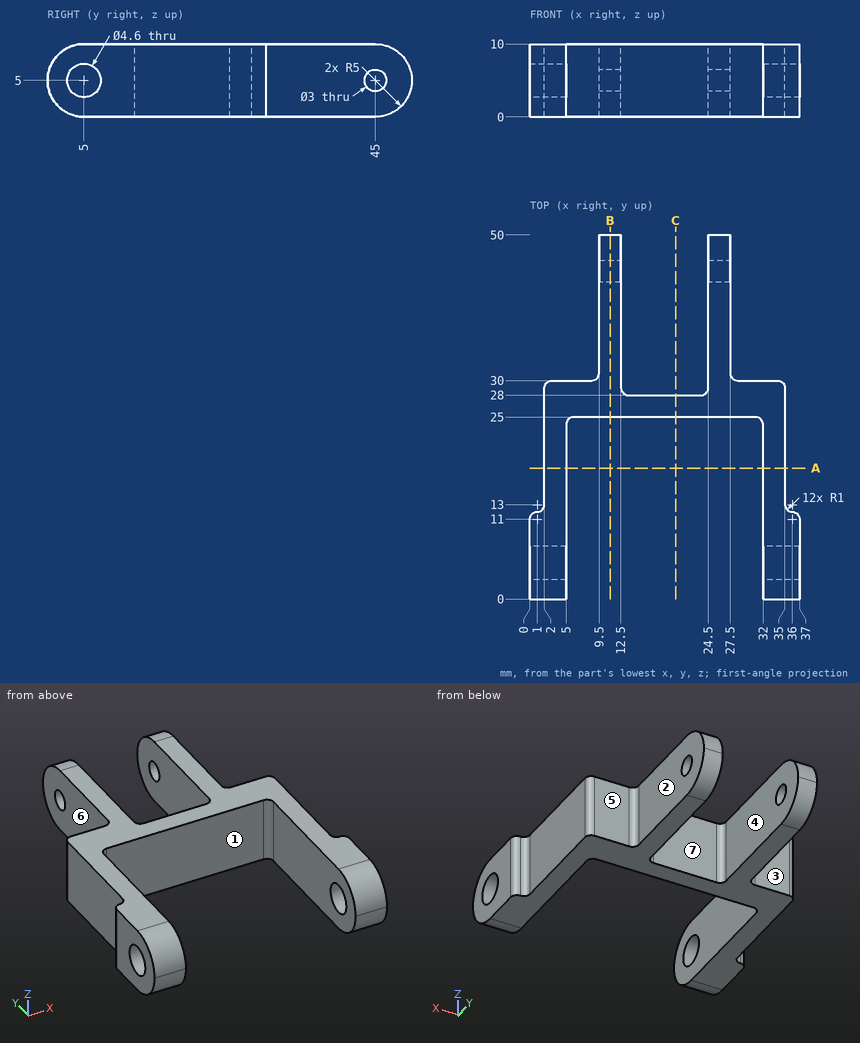
Here's the drawing with two shaded views (mm, measured from the low corner). I have some questions. A direction names the side the tool comes from. Give positions to 0.01 mm unless a question says otherwise; leave off trailing zeros. Write each loop counter-clockwise with the first axis right and the second up, starting at its lowest first coordinate (ties: lowest second). Pieces come first, ordered by that corner, then holes. Notation, with made-up numbers: (45, -25.5) - (49, -25.5) arc R28 ccw to (49, -0.5) - close; hole circle Ø5 at (-19, 34.25). An arc over 180 degrees is marked (long way). Write item = value, one per line. Start each with the question number.
1. On a 3-axis mill with a long thin cutter (end or side, diameter ignored), from which of +Z, -Z, +X, -X, +Y, -Y can I reach the whole of each face in a straight line? I mean the marked faces 1, 2, 3 and 4. Say none if no direction works.
2. Imagine slicing it at A-A (y = 18). Please give me the cut outline in (x, z).
3. Thinking about a two-plate mould opening in X: for the marked faces 5, 6 and 7, which applies, released by +X, released by -X, zero draft, split by the parting line, or undercut?
4. For pin 1 (3 mm diameter, centred on x = 6, z = 6, fed in from +Y); pin 2 (3 mm diameter, centred on y = 17.5, z = 5, fed in from +X); pin 3 (3 mm diameter, centred on x = 19.5, z = 5, fed in from +Y), each with a flat end and sliding along its axis, tell me the tip position at first contact or that it passes through.
5. Please list where these lines run through material, in increasing order: line 1 (X direction, y = 6.5, z = 2.25); line 2 (Z direction, x = 11, y = 45); line 3 (Y direction, x = 25.35, z = 5).
6. Imagine slicing it at C-C (x = 20). Please give me the cut outline in (y, z), and give its area (3 significant figures).
7. Imagine slicing it at B-B (x = 11). Please give me the cut outline in (y, z).
Worked answers:
q1.face_1 = +Z, -Z, -Y
q1.face_2 = +Z, -Z, +X, +Y
q1.face_3 = +Z, -Z, -X, +Y
q1.face_4 = +Z, -Z, +Y
q2.outline = (2, 0) - (5, 0) - (5, 10) - (2, 10) - close; (32, 0) - (35, 0) - (35, 10) - (32, 10) - close
q3.face_5 = zero draft
q3.face_6 = released by -X
q3.face_7 = undercut
q4.pin_1 = 30
q4.pin_2 = 35
q4.pin_3 = 28
q5.line_1 = 0 to 5, 32 to 37
q5.line_2 = 0 to 3.5, 6.5 to 10
q5.line_3 = 25 to 43.5, 46.5 to 50
q6.outline = (25, 0) - (28, 0) - (28, 10) - (25, 10) - close
q6.area = 30.0 mm2
q7.outline = (25, 0) - (45, 0) arc R5 ccw to (45, 10) - (25, 10) - close; hole circle Ø3 at (45, 5)
